Job drawing, mm, ordinate dimensions from the low corner. One solid piece. A direction names the side the tool comes from. Give positions to 0.01 mm unless a question says otherwise; leave off trailing zeros. Order: outer loops, then holes, each group sorted by start corner. A loop starts at its lowest first (then second) coordinate and runs counter-clockwise, first axis right, second up.
1. Probe line 1 (Y direction, x = 6.5, z = 3); line 2 (X direction, y = 7.5, z = 1.5); line 3 (Y direction, x = 2.75, z = 5.25). List the from-to ranges inside material, lowest first.
2. Which spindle directions (+Z, -Z, +X, -X, +Y, -Y) get a long thin tool onto all of the face, cutting with end or side? Do the marked faces 1, 2 and 3. Say none if no direction does.
3. Slice it at A-A on y = 8. List the corners of the cut face in (x, z).
4. Mould opens along Y. For the marked faces 4, 5 and 6 say: +Y half, -Y half, draft (parallel to the pull), parting line (faces both ways), or undercut.
5. Slice it at D-D on z = 2.5. List the corners of the cut face in (x, y), and give its area (3 significant figures).
6. Drop flat-ended pins along their axis: pin 1 Ø1.5 at (y, z) = (14.5, 2.5) entering from +X; pin 2 Ø1 at (y, z) = (3.5, 3) entering from +X; pin 3 Ø1.8 at (y, z) = (6.5, 3) entering from -X. Give the stop position or say it passes through.
7. Slice it at C-C on y = 12. List the corners of the cut face in (x, z), and give its area (3 significant figures).
8. Slice it at B-B on z = 5.25. List the corners of the cut face in (x, y).
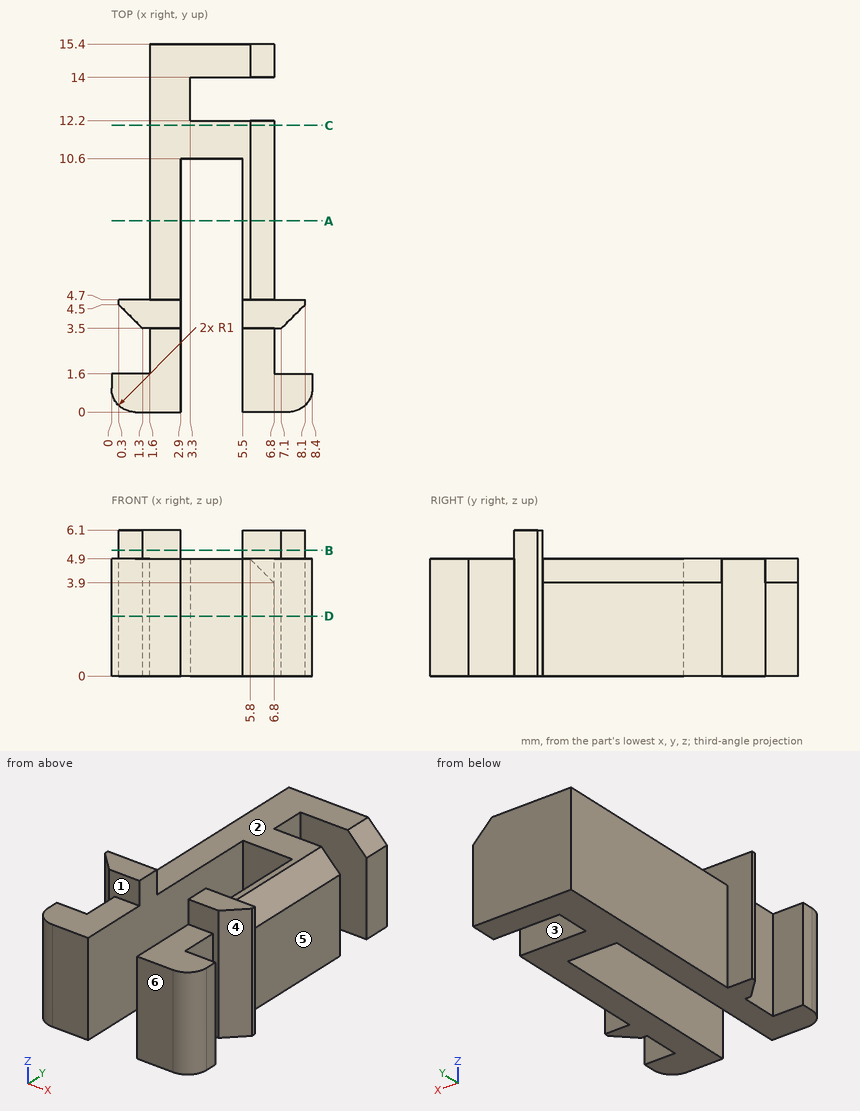
Data:
1. line 1: y = 0 to 12.2, 14 to 15.4
1. line 2: x = 1.6 to 2.9, 5.5 to 6.8
1. line 3: y = 3.5 to 4.7
2. face 1: +Z, -X
2. face 2: +Z, +X, -X, +Y
2. face 3: +Z, -Z, +X
3. outline: (1.6, 0) - (2.9, 0) - (2.9, 4.9) - (1.6, 4.9) - close; (5.5, 0) - (6.8, 0) - (6.8, 3.9) - (5.8, 4.9) - (5.5, 4.9) - close
4. face 4: undercut
4. face 5: draft
4. face 6: -Y half
5. outline: (0, 1) arc R1 ccw to (1, 0) - (2.9, 0) - (2.9, 10.6) - (5.5, 10.6) - (5.5, 0) - (7.4, 0) arc R1 ccw to (8.4, 1) - (8.4, 1.6) - (6.8, 1.6) - (6.8, 3.5) - (7.1, 3.5) - (8.1, 4.5) - (8.1, 4.7) - (6.8, 4.7) - (6.8, 12.2) - (3.3, 12.2) - (3.3, 14) - (6.8, 14) - (6.8, 15.4) - (1.6, 15.4) - (1.6, 4.7) - (0.3, 4.7) - (0.3, 4.5) - (1.3, 3.5) - (1.6, 3.5) - (1.6, 1.6) - (0, 1.6) - close
5. area: 53.0 mm2
6. pin 1: stops at x = 6.8
6. pin 2: stops at x = 7.6
6. pin 3: stops at x = 1.6
7. outline: (1.6, 0) - (6.8, 0) - (6.8, 3.9) - (5.8, 4.9) - (1.6, 4.9) - close
7. area: 25.0 mm2
8. outline: (0.3, 4.5) - (1.3, 3.5) - (2.9, 3.5) - (2.9, 4.7) - (0.3, 4.7) - close; (5.5, 3.5) - (7.1, 3.5) - (8.1, 4.5) - (8.1, 4.7) - (5.5, 4.7) - close
